from build123d import *

# Parameters (mm, degrees)
CROQUIS2_R              = 2
CROQUIS2_W              = 40.4
CROQUIS2_H              = 40
SALIENTE_EXTRUIR1_DEPTH = 5.5
CROQUIS3_W              = 5.5
CROQUIS3_H              = 21
SALIENTE_EXTRUIR2_DEPTH = 2.5
CROQUIS4_W              = 15.5
CROQUIS4_H              = 5.5
CROQUIS4_W_2            = 21
SALIENTE_EXTRUIR3_DEPTH = 2.5
CROQUIS5_W              = 15.5
CROQUIS5_H              = 5.5
CROQUIS5_W_2            = 21
SALIENTE_EXTRUIR4_DEPTH = 2.5


with BuildPart() as part:
    # Croquis2 → Saliente-Extruir1 (new body)
    with BuildSketch(Plane.XY):
        Polygon((-10.5, 50), (-10.5, -34), (42.85, -34), (42.85, -40), (-10.5, -40), (-10.5, -50), (10.5, -50), (10.5, -47), (31.5, -47), (31.5, -50), (47, -50), (47, -31.5), (50, -31.5), (50, -10.5), (47, -10.5), (47, 10.5), (50, 10.5), (50, 31.5), (47, 31.5), (47, 50), (31.5, 50), (31.5, 47), (10.5, 47), (10.5, 50), align=None)
        with Locations((42.85, 5)):
            Circle(CROQUIS2_R, mode=Mode.SUBTRACT)
        with Locations((-5.65, 5)):
            Circle(CROQUIS2_R, mode=Mode.SUBTRACT)
        with Locations((42.85, -5)):
            Circle(CROQUIS2_R, mode=Mode.SUBTRACT)
        with Locations((-5.65, -5)):
            Circle(CROQUIS2_R, mode=Mode.SUBTRACT)
        with Locations((18.5, 0)):
            Rectangle(CROQUIS2_W, CROQUIS2_H, mode=Mode.SUBTRACT)
    extrude(amount=SALIENTE_EXTRUIR1_DEPTH)

    # Croquis3 → Saliente-Extruir2 (add)
    with BuildSketch(Plane(origin=(50, 0, 0), x_dir=(0, 0, -1), z_dir=(1, 0, 0))):
        with Locations((-2.75, -21)):
            Rectangle(CROQUIS3_W, CROQUIS3_H)
        with Locations((-2.75, 21)):
            Rectangle(CROQUIS3_W, CROQUIS3_H)
    extrude(amount=SALIENTE_EXTRUIR2_DEPTH)

    # Croquis4 → Saliente-Extruir3 (add)
    with BuildSketch(Plane(origin=(0, 50, 0), x_dir=(1, 0, 0), z_dir=(0, 1, 0))):
        with Locations((39.25, -2.75)):
            Rectangle(CROQUIS4_W, CROQUIS4_H)
        with Locations((0, -2.75)):
            Rectangle(CROQUIS4_W_2, CROQUIS4_H)
    extrude(amount=SALIENTE_EXTRUIR3_DEPTH)

    # Croquis5 → Saliente-Extruir4 (add)
    with BuildSketch(Plane.XZ.offset(50)):
        with Locations((39.25, 2.75)):
            Rectangle(CROQUIS5_W, CROQUIS5_H)
        with Locations((0, 2.75)):
            Rectangle(CROQUIS5_W_2, CROQUIS5_H)
    extrude(amount=SALIENTE_EXTRUIR4_DEPTH)


solid = part.part
The listing builds one solid part. Answer for the finished solid, in the listing's coordinates (mm). A direction names the side the tool comes from. Round coordinates to 2 decimals unless told otherwise and drop trailing zeros. Order: outer loops, then holes, each group sorted by start corner. A loop starts at its lowest first (then second) coordinate and runs counter-clockwise, first axis right, second up. Notation, with made-up numbers: (64.5, -26.5) -> (121.5, -26.5) arc R16 ccw to (121.5, -8.5) -> close; hole circle Ø2 at (-19, 72). An arc over 180 degrees is marked (long way). Write each question's results on one line, items separated by ' | '. Start each with the question number.
Q1. The mould has two halves that part along Y. Classify faces 1 (the flat face through (18, -20, 3)), 2 (the flat face through (38.7, 0, 3)), 3 (the flat face through (39, -52.5, 3)), 4 (the flat face through (21, 24, 0)): pulls with the +Y half, pulls with the -Y half, needs draft (parallel to the pull), parting line crosses it, or undercut.
Q2. Find section C-C (z = 2.6). Give the number of separate pieces and of enclosed holes in the cut face, then the cut area to 3 significant figures.
Q3. Each of these flat-tipped pins is pushed along its axis until it touches: pin 1 (1.6 mm diameter, centred on y = 50, z = 4, fed in from +X); pin 2 (3 mm diameter, centred on x = 23.5, z = 4, fed in from +Y). Where does it stop, or does it pass through?
Q4. Find section B-B (x = -5.65). Determine the outline of the cut face in (y, z), then the cut area to 4 significant figures.
Q5. Straight lines are drawn through the part: probe 1 along Y at (x, z) = (30, 3.5); probe 2 along Y at (x, z) = (-5.65, 3.3); probe 3 along Y at (x, z) = (10, 2.7). For each, find the intervals that lie inside material, in ascending order. Write a range as from..to.
Q6. Find section D-D (x = 13). Determine the outline of the cut face in (y, z).
Q7. Find section A-A (y = -5). Determine the outline of the cut face in (x, z).
Q8. Which of the six approach directions +Z, -Z, +X, -X, +Y, -Y give full straight-line access (tool end or side, diameter ignored) to faces 5 (the flat face through (10.5, -50, 3)), 6 (the flat face through (21, 47, 3)), 7 (the flat face through (16, -34, 3)), 8 (the flat face through (-1.7, 0, 3)), 9 (the flat face through (50, 10.5, 3))?
Worked answers:
1) face 1: undercut | face 2: undercut | face 3: pulls with the -Y half | face 4: needs draft
2) separate pieces: 1 | enclosed holes: 5 | area: 4,050 mm2
3) pin 1: stops at x = 47 | pin 2: stops at y = 47
4) outline: (-52.5, 0) -> (-40, 0) -> (-40, 5.5) -> (-52.5, 5.5) -> close; (-34, 0) -> (-7, 0) -> (-7, 5.5) -> (-34, 5.5) -> close; (-3, 0) -> (3, 0) -> (3, 5.5) -> (-3, 5.5) -> close; (7, 0) -> (52.5, 0) -> (52.5, 5.5) -> (7, 5.5) -> close | area: 500.5 mm2
5) probe 1: y = -47..-40, -34..-20, 20..47 | probe 2: y = -52.5..-40, -34..-7, -3..3, 7..52.5 | probe 3: y = -52.5..-40, -34..-20, 20..52.5
6) outline: (-47, 0) -> (-40, 0) -> (-40, 5.5) -> (-47, 5.5) -> close; (-34, 0) -> (-20, 0) -> (-20, 5.5) -> (-34, 5.5) -> close; (20, 0) -> (47, 0) -> (47, 5.5) -> (20, 5.5) -> close
7) outline: (-10.5, 0) -> (-7.65, 0) -> (-7.65, 5.5) -> (-10.5, 5.5) -> close; (-3.65, 0) -> (-1.7, 0) -> (-1.7, 5.5) -> (-3.65, 5.5) -> close; (38.7, 0) -> (40.85, 0) -> (40.85, 5.5) -> (38.7, 5.5) -> close; (44.85, 0) -> (47, 0) -> (47, 5.5) -> (44.85, 5.5) -> close
8) face 5: +Z, -Z, -Y | face 6: +Z, -Z, +Y | face 7: +Z, -Z, -X | face 8: +Z, -Z | face 9: +Z, -Z, +X
